```python
from build123d import *

# Parameters (mm, degrees)
CROQUIS1_R              = 4.5
SALIENTE_EXTRUIR1_DEPTH = 6
CROQUIS2_W              = 120
CROQUIS2_H              = 6
SALIENTE_EXTRUIR2_DEPTH = 186
CROQUIS3_W              = 120
CROQUIS3_H              = 44
SALIENTE_EXTRUIR3_DEPTH = 6
REDONDEO1_R             = 10
CROQUIS4_R              = 2.621
CORTAR_EXTRUIR1_DEPTH   = 259.417772547


with BuildPart() as part:
    # Croquis1 → Saliente-Extruir1 (new body)
    with BuildSketch(Plane.XY):
        Polygon((-92.102036721, -168.3), (-57.102036721, -244.5), (-7.102036721, -244.5), (27.897963279, -168.3), (27.897963279, -92.1), (-92.102036721, -92.1), align=None)
        with Locations((-83.602036721, -111.15)):
            Circle(CROQUIS1_R, mode=Mode.SUBTRACT)
        with Locations(Location((-83.602036721, -149.25, 0), (0, 0, 180))):
            Circle(CROQUIS1_R, mode=Mode.SUBTRACT)
        with Locations((19.397963279, -149.25)):
            Circle(CROQUIS1_R, mode=Mode.SUBTRACT)
        with Locations(Location((19.397963279, -111.15, 0), (0, 0, 180))):
            Circle(CROQUIS1_R, mode=Mode.SUBTRACT)
    extrude(amount=SALIENTE_EXTRUIR1_DEPTH)

    # Croquis2 → Saliente-Extruir2 (add)
    with BuildSketch(Plane.XY.offset(6)):
        with Locations((-32.102036721, -95.1)):
            Rectangle(CROQUIS2_W, CROQUIS2_H)
    extrude(amount=SALIENTE_EXTRUIR2_DEPTH)

    # Croquis3 → Saliente-Extruir3 (add)
    with BuildSketch(Plane.XY.offset(192)):
        with Locations((-32.102036721, -120.1)):
            Rectangle(CROQUIS3_W, CROQUIS3_H)
    extrude(amount=-SALIENTE_EXTRUIR3_DEPTH)

    # Redondeo1
    redondeo1_edges = [part.edges().sort_by_distance(p)[0] for p in [
        (27.897963279, -168.3, 3),
        (-7.102036721, -244.5, 3),
        (-57.102036721, -244.5, 3),
        (-92.102036721, -168.3, 3),
        (-32.102036721, -92.1, 192),
        (-92.102036721, -142.1, 189),
        (-32.102036721, -98.1, 186),
        (27.897963279, -142.1, 189),
        (-32.102036721, -92.1, 0),
    ]]
    fillet(redondeo1_edges, radius=REDONDEO1_R)

    # Croquis4 → Cortar-Extruir1 (cut, through all)
    with BuildSketch(Plane.XZ.offset(98.1)):
        with Locations(Location((1.485535385, 83.587572106, 0), (0, 0, 270))):
            Circle(CROQUIS4_R)
        with Locations(Location((-65.689608828, 16.412427894, 0), (0, 0, 270))):
            Circle(CROQUIS4_R)
        with Locations(Location((15.397963279, 50, 0), (0, 0, 270))):
            Circle(CROQUIS4_R)
        with Locations(Location((1.485535385, 16.412427894, 0), (0, 0, 270))):
            Circle(CROQUIS4_R)
        with Locations(Location((-65.689608828, 83.587572106, 0), (0, 0, 270))):
            Circle(CROQUIS4_R)
        with Locations(Location((-32.102036721, 97.5, 0), (0, 0, 270))):
            Circle(CROQUIS4_R)
        with Locations(Location((-79.602036721, 50, 0), (0, 0, 270))):
            Circle(CROQUIS4_R)
        with BuildLine():
            add(Edge.make_bspline(
                [(-32.102036721, 6.5), (-30.775341976, 6.499993534), (-28.122039283, 6.620682339), (-24.096613371, 7.177840976), (-20.062551193, 8.127248902), (-16.009319538, 9.510205402), (-12.057431762, 11.308759473), (-8.231122582, 13.545008905), (-4.625202085, 16.175326085), (-1.288566333, 19.186782917), (1.722751008, 22.523306389), (4.353148795, 26.129382286), (6.589284057, 29.95555323), (8.387887512, 33.907608072), (9.770762576, 37.960684071), (10.720181934, 41.994878278), (11.277273839, 46.020137925), (11.45831212, 50.000176972), (11.277257351, 53.980039938), (10.720117639, 58.005467444), (9.770712855, 62.03948534), (8.387758304, 66.092717236), (6.589203689, 70.044604944), (4.352954406, 73.870914143), (1.722637185, 77.476834635), (-1.288819636, 80.813470389), (-4.62534311, 83.824787729), (-8.231419007, 86.455185516), (-12.057589951, 88.691320778), (-16.009644794, 90.489924234), (-20.062720792, 91.872799297), (-24.096914999, 92.822218655), (-28.122174647, 93.37931056), (-32.102213693, 93.560348842), (-36.082076659, 93.379294072), (-40.107504165, 92.82215436), (-44.141522061, 91.872749576), (-48.194753957, 90.489795025), (-52.146641666, 88.691240411), (-55.972950865, 86.454991127), (-59.578871356, 83.824673906), (-62.91550711, 80.813217085), (-65.92682445, 77.476693611), (-68.557222237, 73.870617714), (-70.7933575, 70.04444677), (-72.591960955, 66.092391928), (-73.974836018, 62.039315929), (-74.924255376, 58.005121722), (-75.481347281, 53.979862075), (-75.662385563, 49.999823028), (-75.481330794, 46.019960062), (-74.924191081, 41.994532556), (-73.974786297, 37.96051466), (-72.591831746, 33.907282764), (-70.793277132, 29.955395056), (-68.557027848, 26.129085856), (-65.926710628, 22.523165366), (-62.915253807, 19.186529609), (-59.578730331, 16.17521228), (-55.972654439, 13.544814452), (-52.146483477, 11.308679338), (-48.194428701, 9.51007534), (-44.141352462, 8.127202224), (-40.107202532, 7.177786011), (-36.081941291, 6.620713021), (-33.428642641, 6.500006466), (-32.102036721, 6.5)],
                knots=[0, 0, 0, 0, 0.014562552, 0.029124133, 0.044561437, 0.059996822, 0.076077508, 0.092156266, 0.108579119, 0.125000004, 0.141422857, 0.157843742, 0.173924427, 0.190003186, 0.20544049, 0.220875875, 0.235438912, 0.250000004, 0.264563041, 0.279124133, 0.294561437, 0.309996822, 0.326077508, 0.342156266, 0.358579119, 0.375000004, 0.391422857, 0.407843742, 0.423924427, 0.440003186, 0.45544049, 0.470875875, 0.485438912, 0.500000004, 0.514563041, 0.529124133, 0.544561437, 0.559996822, 0.576077508, 0.592156266, 0.608579119, 0.625000004, 0.641422857, 0.657843742, 0.673924427, 0.690003186, 0.70544049, 0.720875875, 0.735438912, 0.750000004, 0.764563041, 0.779124133, 0.794561437, 0.809996822, 0.826077508, 0.842156266, 0.858579119, 0.875000004, 0.891422857, 0.907843742, 0.923924427, 0.940003186, 0.95544049, 0.970875875, 0.985438423, 1, 1, 1, 1], degree=3))
        make_face()
    extrude(amount=-CORTAR_EXTRUIR1_DEPTH, mode=Mode.SUBTRACT)


solid = part.part
```
Geometry check sheet. Reference: the model listing, model coordinates, mm. A direction names the side the tool comes from. Coordinates: 2 decimals unless noted, no trailing zeros. Loops run counter-clockwise (first coordinate to the right, second up) from the corner with the lowest first, then second, coordinate; pieces in that order, holes last. Notation, with made-up numbers: (-18.75, 25) - (31.25, 25) arc R31 cw to (31.25, 63) - close; hole circle Ø10 at (14.5, 12.5). An arc over 180 degrees is marked (long way). One line per item, written item: value. Start each with the question number.
(1) Cross-section at C-C on y = -111.15. Enter the section's corners in (x, z), plus the area to 3 significant figures.
(2) Cross-section at A-A on z = 97.5. Enter the section's corners in (x, y).
(3) Material ranges on line 1 (Z direction, x = -5.5, y = -142); line 2 (Y direction, x = -82.5, z = 112.5); line 3 (X direction, y = -95.15, z = 97.5), recorded low to high. Write a range as [from, to].
(4) Depth check by flat-ended pin: P1, Ø4, axis at x = -65.69, z = 16.41, coming from the +Y side; P2, Ø5.5, axis at x = -83.6, y = -111.15, coming from the -Z side; P3, Ø6, axis at x = -74.5, y = -191.5, coming from the +Z side; P4, Ø12, axis at x = -1.5, z = 116, coming from the -Y side. Enter the tip coordinate at first touch or a pass-through.
(5) Cross-section at B-B on y = -149.25. Enter the section's corners in (x, z), plus the area to 3 significant figures.
(6) Cross-section at D-D on y = -128.5. Enter the section's corners in (x, z), plus the area to 3 significant figures.
(7) Tool access check on faces 1 (the flat face through (-33, -170, 6)), 2 (the cylindrical face through (-89.25, -139.093, 188.958)), 3 (the cylindrical face through (19.984, -115.612, 2.958)), 4 (the flat face through (-33, -142.1, 189)). Record the directions out of +Z, -Z, +X, -X, +Y, -Y that give a thin tool (end or side, any length) a straight path to the whole face; none if there is none.
(8) Mould release check, pull along Z, two halves, no side actions. Record for faces 5 (the cylindrical face through (-56.02, -242.96, 3.04)), 6 (the cylindrical face through (-81.927, -95.142, 48.791)): released by +Z, released by -Z, zero draft, split by the parting line, or undercut.
Results below:
1. outline: (-92.1, 0) - (-88.1, 0) - (-88.1, 6) - (-92.1, 6) - close; (-92.1, 186) - (27.9, 186) - (27.9, 192) - (-92.1, 192) - close; (-79.1, 0) - (14.9, 0) - (14.9, 6) - (-79.1, 6) - close; (23.9, 0) - (27.9, 0) - (27.9, 6) - (23.9, 6) - close
1. area: 1,330 mm2
2. outline: (-92.1, -98.1) - (-34.72, -98.1) - (-34.72, -92.1) - (-92.1, -92.1) - close; (-29.48, -98.1) - (27.9, -98.1) - (27.9, -92.1) - (-29.48, -92.1) - close
3. line 1: z = [0, 6], [186, 192]
3. line 2: y = [-98.1, -92.1]
3. line 3: x = [-92.1, -34.72], [-29.48, 27.9]
4. P1: passes through
4. P2: stops at z = 186
4. P3: stops at z = 6
4. P4: stops at y = -98.1
5. outline: (-92.1, 0) - (-88.1, 0) - (-88.1, 6) - (-92.1, 6) - close; (-79.1, 0) - (14.9, 0) - (14.9, 6) - (-79.1, 6) - close; (23.9, 0) - (27.9, 0) - (27.9, 6) - (23.9, 6) - close
5. area: 612 mm2
6. outline: (-92.1, 0) - (27.9, 0) - (27.9, 6) - (-92.1, 6) - close; (-92.1, 186) - (27.9, 186) - (27.9, 192) - (-92.1, 192) - close
6. area: 1,440 mm2
7. face 1: +X, -X, -Y
7. face 2: +Z, -X, -Y
7. face 3: -Z
7. face 4: +Z, +X, -X, -Y
8. face 5: zero draft
8. face 6: undercut
